Autodesk Inventor part; units mm, degrees
ref_plane "YZ Plane" through (0, 0, 0) normal (1, 0, 0) x (0, 1, 0)
ref_plane "XZ Plane" through (0, 0, 0) normal (0, 1, 0) x (-1, 0, 0)
ref_plane "XY Plane" through (0, 0, 0) normal (0, 0, 1) x (1, 0, 0)
sketch "Эскиз1" plane through (0, 0, 0) normal (0, 1, 0) x (-1, 0, 0)
  line L0 (6.5, 22) -> (-6.5, 22)
  line L1 (-6.5, 22) -> (-6.5, -22)
  line L2 (-6.5, -22) -> (6.5, -22)
  line L3 (6.5, -22) -> (6.5, 22)
  line L4 (-6.5, 22) -> (6.5, -22) construction
  line L5 (0, 22) -> (0, -22) construction
  circle A0 centre (0, 16) radius 2
  line L6 (6.5, 0) -> (-6.5, 0) construction
  circle A1 centre (0, -16) radius 2
  point P0 (0, 0)
  point P1 (0, 0)
  dimension "d0" = 13
  dimension "d1" = 44
  dimension "d2" = 16
  dimension "d3" = 4
extrude "Выдавливание1" add sketch "Эскиз1" along normal blind 32
sketch "Эскиз2" plane through (6.5, 0, 22) normal (1, 0, 0) x (0, 0, -1)
  line L0 (0, 32) -> (44, 32)
  line L1 (44, 0) -> (0, 0)
  line L2 (44, 32) -> (0, 0) construction
  circle A0 centre (22, 16) radius 10.15
  line L3 (11.85, 16) -> (32.15, 16) construction
  circle A1 centre (14.5, 16) radius 1.15
  circle A2 centre (29.5, 16) radius 1.15
  line L4 (14.5, 16) -> (29.5, 16)
  circle A3 centre (22, 16) radius 13.15
  line L5 (22, 29.15) -> (22, 2.85)
  line L6 (44, 0) -> (44, 32)
  circle A4 centre (22, 16) radius 3.65
  point P0 (22, 0)
  dimension "d9" = 20.3
  dimension "d10" = 2.3
  dimension "d11" = 15
  dimension "d17" = 7.3
  dimension "d21" = 26.3
extrude "Выдавливание3" cut sketch "Эскиз2" against normal through all contours A2 | A1 | A4 L4 L5 | L5 L4 A4 | A4 L4 L5 | L5 L4 A4
extrude "Выдавливание4" cut sketch "Эскиз2" against normal blind 9
ref_plane "РабПлоскость1" through (0, 25, 0) normal (0, 1, 0) x (1, 0, 0)
sketch "Эскиз3" plane through (0, 25, 0) normal (0, 1, 0) x (1, 0, 0)
  circle A0 centre (0, -16) radius 2
  circle A1 centre (0, 16) radius 2
  point P0 (0, 0)
extrude "Выдавливание5" add sketch "Эскиз3" against normal blind 16
fillet "Сопряжение1" radius 6 2 edges at (6.5, 16, 22) (6.5, 16, -22)
chamfer "Фаска1" distance 1.2 angle 45 2 edges at (-6.5, 16, -6.35) (-6.5, 16, 8.65)
properties part number "motor_mount_edge"
Can you work these out from the model? Positions are in its coordinate system, mm. A direction names the side the tool comes from. Coordinates: 2 decimals unless noted, no trailing zeros. Loops run counter-clockwise (first coordinate to the right, second up) from the corner with the lowest first, then second, coordinate; pieces in that order, holes last. Notation, with made-up numbers: (51.5, -38.5) -> (55.5, -38.5) arc R27 cw to (55.5, -8.5) -> close; hole circle Ø4 at (47, -36.5). An arc over 180 degrees is marked (long way). Answer as a JSON object with one key per item and string values.
1) If I drill on line 1 (Y direction, x = 1.75, z = 0); line 2 (Z direction, x = -1.5, y = 28); line 3 (Y direction, x = -3.2, z = 7.5), over which ranges is the centre line in solid material (lowest first)?
Results:
{"line 1": "y = 0 to 2.85, 29.15 to 32", "line 2": "z = -22 to -17.32, -14.68 to -5.38, 5.38 to 14.68, 17.32 to 22", "line 3": "y = 0 to 14.85, 17.15 to 32"}
2) For P1, Ø1.2, axis at x = 0.5, z = 16.5, coming from the +Y side; P2, Ø3, axis at y = 16, z = 7.5, coming from the +X side; P3, Ø1.5, axis at x = 3, y = 18.5, coming from the +Z side, each with a flat end and sliding along its axis, tell me the tip position at first contact or that it passes through.
Results:
{"P1": "stops at y = 25", "P2": "stops at x = -2.5", "P3": "stops at z = 21.74"}
3) Imagine slicing it at C-C (y = 4.5). Please give me the cut outline in (x, z), then the cut area to 3 significant figures.
Results:
{"outline": "(-6.5, -22) -> (0.5, -22) arc R6 ccw to (6.5, -16) -> (6.5, -6.38) -> (-2.5, -6.38) -> (-2.5, 6.38) -> (6.5, 6.38) -> (6.5, 16) arc R6 ccw to (0.5, 22) -> (-6.5, 22) -> close; hole circle Ø4 at (0, -16); hole circle Ø4 at (0, 16)", "area": "417 mm^2"}
4) Imagine slicing it at B-B (x = 0). Please give me the cut outline in (y, z).
Results:
{"outline": "(0, -22) -> (32, -22) -> (32, -18) -> (25, -18) -> (25, -14) -> (32, -14) -> (32, 14) -> (25, 14) -> (25, 18) -> (32, 18) -> (32, 22) -> (0, 22) -> (0, 18) -> (9, 18) -> (9, 14) -> (0, 14) -> (0, -14) -> (9, -14) -> (9, -18) -> (0, -18) -> close; hole circle Ø26.3 at (16, 0)"}
5) Imagine slicing it at D-D (z = -7.5). Please give me the cut outline in (x, y), then the cut area to 3 significant figures.
Results:
{"outline": "(-6.5, 0) -> (6.5, 0) -> (6.5, 5.2) -> (-2.5, 5.2) -> (-2.5, 14.85) -> (-5.3, 14.85) -> (-6.5, 13.65) -> close; (-6.5, 18.35) -> (-5.3, 17.15) -> (-2.5, 17.15) -> (-2.5, 26.8) -> (6.5, 26.8) -> (6.5, 32) -> (-6.5, 32) -> close", "area": "211 mm^2"}
6) Imagine slicing it at A-A (y = 16). Please give me the cut outline in (x, z).
Results:
{"outline": "(-6.5, -22) -> (0.5, -22) arc R6 ccw to (6.5, -16) -> (6.5, -13.15) -> (-2.5, -13.15) -> (-2.5, -8.65) -> (-5.3, -8.65) -> (-6.5, -9.85) -> close; (-6.5, -5.15) -> (-5.3, -6.35) -> (-2.5, -6.35) -> (-2.5, -3.65) -> (-6.5, -3.65) -> close; (-6.5, 3.65) -> (-2.5, 3.65) -> (-2.5, 6.35) -> (-5.3, 6.35) -> (-6.5, 5.15) -> close; (-6.5, 9.85) -> (-5.3, 8.65) -> (-2.5, 8.65) -> (-2.5, 13.15) -> (6.5, 13.15) -> (6.5, 16) arc R6 ccw to (0.5, 22) -> (-6.5, 22) -> close"}
7) For faces 1 (the face through (2.063, 3.163, 2.851)), 2 (the face through (-3.88, 14.98, -8.03)), 3 (the face through (0, 28, 14)), 4 (the face through (0, 4, 14)), which set-ups out of +Z, -Z, +X, -X, +Y, -Y let a thin tool reach every point of the face, with its end or its side?
Results:
{"face 1": "+X", "face 2": "+X, -X", "face 3": "+Y", "face 4": "-Y"}
8) Thinking about a two-plate mould opening in Y: for faces 5 (the face through (0, 28, -18)), 6 (the face through (-4.47, 19.08, -1.96)), 7 (the face through (0, 32, 0)), which applies, pulls with the +Y half, pulls with the -Y half, needs draft (parallel to the pull), parting line crosses it, or undercut?
Results:
{"face 5": "needs draft", "face 6": "undercut", "face 7": "pulls with the +Y half"}
